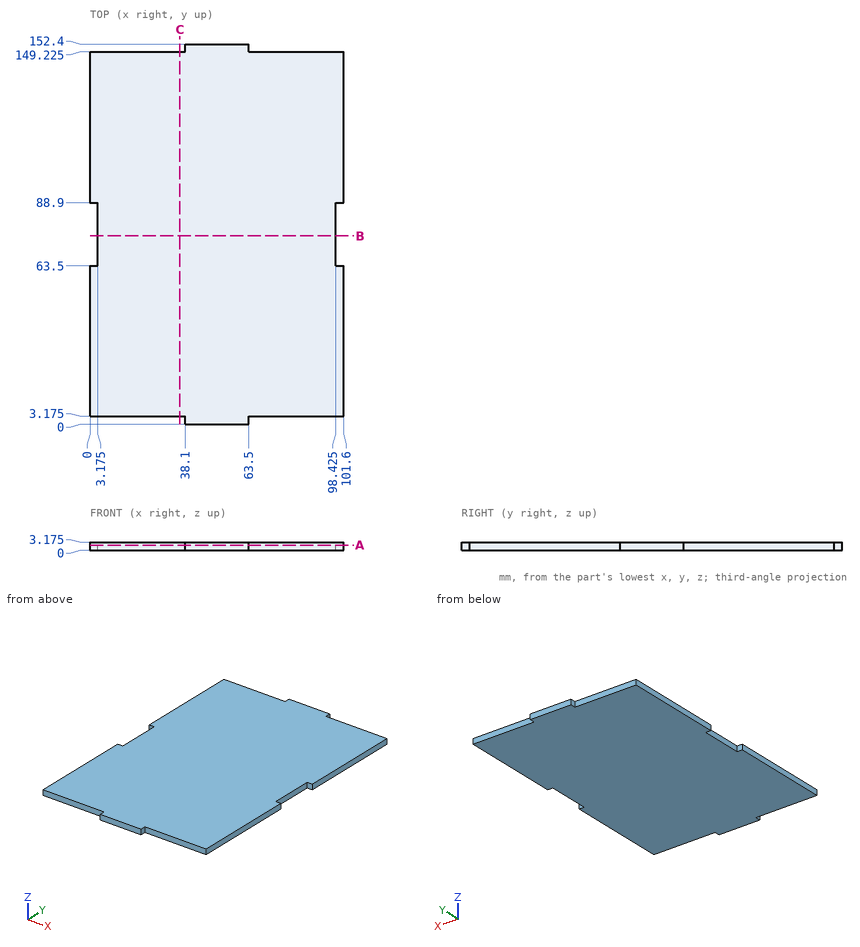
Here's the drawing with two shaded views (mm, measured from the low corner). I have some questions. Coordinates: 2 decimals unless noted, no trailing zeros. Order: outer loops, then holes, each group sorted by start corner. A loop starts at its lowest first (then second) coordinate and runs counter-clockwise, first axis right, second up. Notation, with made-up numbers: (-13.75, -39.5) - (17.25, -39.5) arc R25 ccw to (17.25, -19.5) - close; hole circle Ø3 at (-31.5, 26.25). An arc over 180 degrees is marked (long way). Use CSV: the item, a comma, the result in double quotes. Start each with the question number.
1. Suppose I cut it at A-A on z = 2.05. List the corners of the cut face in (x, y) for me (3 decimals).
2. Suppose I cut it at B-B on y = 75.5. List the corners of the cut face in (x, z) for me (3 decimals), then the cut area to 3 significant figures.
3. Suppose I cut it at C-C on x = 36. List the corners of the cut face in (y, z) for me (3 decimals), then the cut area to 3 significant figures.
4. I'm going to push flat-ended pins straight in: pin 1 (1 mm diameter, centred on y = 74.5, z = 1.5, fed in from -X) (3 decimals); pin 2 (1.6 mm diameter, centred on y = 77, z = 2.5, fed in from +X) (3 decimals); pin 3 (1.6 mm diameter, centred on x = 87, z = 1.5, fed in from -Y) (3 decimals). Where does each tip first touch, or does it pass through?
5. Please list where these lines run through material, in increasing order: line 1 (X direction, y = 88, z = 1.4) (3 decimals); line 2 (Y direction, x = 71.5, z = 2.85) (3 decimals). Write a range as from..to.
Output:
1,outline,"(0, 3.175) - (38.1, 3.175) - (38.1, 0) - (63.5, 0) - (63.5, 3.175) - (101.6, 3.175) - (101.6, 63.5) - (98.425, 63.5) - (98.425, 88.9) - (101.6, 88.9) - (101.6, 149.225) - (63.5, 149.225) - (63.5, 152.4) - (38.1, 152.4) - (38.1, 149.225) - (0, 149.225) - (0, 88.9) - (3.175, 88.9) - (3.175, 63.5) - (0, 63.5) - close"
2,outline,"(3.175, 0) - (98.425, 0) - (98.425, 3.175) - (3.175, 3.175) - close"
2,area,"302 mm2"
3,outline,"(3.175, 0) - (149.225, 0) - (149.225, 3.175) - (3.175, 3.175) - close"
3,area,"464 mm2"
4,pin 1,"stops at x = 3.175"
4,pin 2,"stops at x = 98.425"
4,pin 3,"stops at y = 3.175"
5,line 1,"x = 3.175..98.425"
5,line 2,"y = 3.175..149.225"
